Can you work these out from the drawing? Everything is in mm from the part's minimum corner. A direction names the side the tool comes from. Coordinates: 2 decimals unless noted, no trailing zeros. Write each loop counter-clockwise with the first axis right and the second up, starting at its lowest first coordinate (ties: lowest second). Pieces come first, ordered by that corner, then holes. Notation, with made-up numbers: (17, 40) -> (43, 40) arc R21 cw to (43, 76) -> close; hole circle Ø7 at (-2, 89). An arc over 180 degrees is marked (long way). Use a Markdown table: item, result. Add a question column.
Item 1: Imagine slicing it at A-A, the plane x = 30. Write out the boundary of the cut face in (y, z), and give its area (3 significant figures).
Item 2: Imagine slicing it at D-D, the plane y = 67. Write out the boundary of the cut face in (x, z).
Item 3: On a 3-axis mill with a long thin cutter (end or side, diameter ignored), from which of +Z, -Z, +X, -X, +Y, -Y can I reach the whole of each face in a straight line? I mean the marked faces 1, 2 and 3. Say none if no direction works.
Item 4: If I drill on line 1 along Y through (x, z) = (14, 21); line 2 along Y through (x, z) = (37, 32); line 3 along Z through (x, y) = (25, 70), over which ranges is the centre line in solid material (lowest first)? Write a range as from..to.
Item 5: Will these pins go through, and if not, where does the flat tip stop? pin 1 Ø2 at (y, z) = (99.5, 37) entering from +X; pin 2 Ø1.5 at (x, z) = (34.5, 26) entering from -Y; pin 3 Ø8 at (y, z) = (62.5, 26) entering from -X.
Item 6: Imagine slicing it at B-B, the plane z = 30. Write out the boundary of the cut face in (x, y).
Item 7: Imagine slicing it at C-C, the plane y = 27.5. Write out the boundary of the cut face in (x, z).
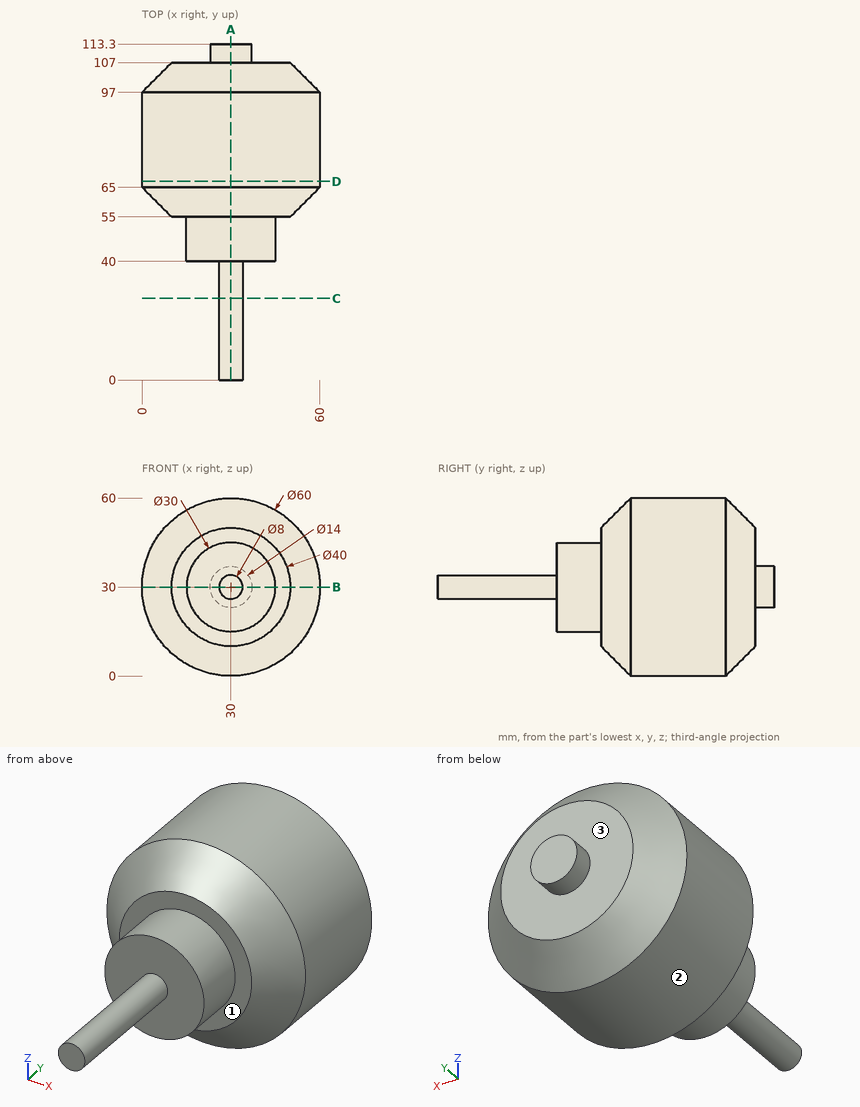
Ans:
| question | item | result |
|---|---|---|
| 1 | outline | (0, 26) -> (40, 26) -> (40, 15) -> (55, 15) -> (55, 10) -> (65, 0) -> (97, 0) -> (107, 10) -> (107, 23) -> (113.3, 23) -> (113.3, 37) -> (107, 37) -> (107, 50) -> (97, 60) -> (65, 60) -> (55, 50) -> (55, 45) -> (40, 45) -> (40, 34) -> (0, 34) -> close |
| 1 | area | 3,780 mm^2 |
| 2 | outline | circle Ø60 at (30, 30) |
| 3 | face 1 | -Y |
| 3 | face 2 | +Y, -Y |
| 3 | face 3 | +Y |
| 4 | line 1 | y = 55..107 |
| 4 | line 2 | y = 40..107 |
| 4 | line 3 | z = 0.42..59.58 |
| 5 | pin 1 | stops at x = 57.66 |
| 5 | pin 2 | stops at y = 40 |
| 5 | pin 3 | stops at x = 0.01 |
| 6 | outline | (0, 65) -> (10, 55) -> (15, 55) -> (15, 40) -> (26, 40) -> (26, 0) -> (34, 0) -> (34, 40) -> (45, 40) -> (45, 55) -> (50, 55) -> (60, 65) -> (60, 97) -> (50, 107) -> (37, 107) -> (37, 113.3) -> (23, 113.3) -> (23, 107) -> (10, 107) -> (0, 97) -> close |
| 7 | outline | circle Ø8 at (30, 30) |
